Work out the finished part from the listing and answer in its coordinate system (mm). A direction names the side the tool comes from. Round coordinates to 2 decimals unless told otherwise and drop trailing zeros. Order: outer loops, then holes, each group sorted by start corner. A loop starts at its lowest first (then second) coordinate and runs counter-clockwise, first axis right, second up. Notation, with made-up numbers: (71, -30.75) - (124, -30.75) arc R24 ccw to (124, 0.25) - close; hole circle Ø10 at (10.5, -14). An arc over 180 degrees is marked (long way). Put each result on its own line as item: value.
Autodesk Inventor part; units mm, degrees
ref_plane "YZ Plane" through (0, 0, 0) normal (1, 0, 0) x (0, 1, 0)
ref_plane "XZ Plane" through (0, 0, 0) normal (0, 1, 0) x (-1, 0, 0)
ref_plane "XY Plane" through (0, 0, 0) normal (0, 0, 1) x (1, 0, 0)
sketch "Sketch1" plane through (0, 0, 0) normal (0, 1, 0) x (-1, 0, 0)
  line L0 (0, 0) -> (-127, 0)
  line L1 (-127, 0) -> (-127, -6.35)
  line L2 (-127, -6.35) -> (0, -6.35)
  line L3 (0, -6.35) -> (0, 0)
  line L4 (0, -6.35) -> (-6.35, -6.35)
  line L5 (-6.35, -6.35) -> (-6.35, -127)
  line L6 (-6.35, -127) -> (0, -127)
  line L7 (0, -127) -> (0, -6.35)
  line L8 (-127, -6.35) -> (-120.65, -6.35)
  line L9 (-120.65, -6.35) -> (-120.65, -127)
  line L10 (-120.65, -127) -> (-127, -127)
  line L11 (-127, -127) -> (-127, -6.35)
  dimension "d0" = 127
  dimension "d1" = 6.35
  dimension "d2" = 6.35
  dimension "d3" = 120.65
  dimension "d4" = 120.65
  dimension "d5" = 6.35
extrude "Extrusion1" add sketch "Sketch1" along normal blind 6.35
sketch "Sketch2" plane through (127, 0, 0) normal (1, 0, 0) x (0, 0, -1)
  line L0 (127, 6.35) -> (120.65, 0)
  line L1 (6.35, 0) -> (127, 0)
  line L2 (127, 0) -> (127, 6.35)
  line L3 (120.65, 0) -> (127, 0)
  line L4 (127, 0) -> (127, 6.35)
  line L5 (127, 6.35) -> (127, 0)
  point P0 (0, 0)
  dimension "d8" = 135
extrude "Extrusion2" cut sketch "Sketch2" against normal blind 152.4
sketch "Sketch4" plane through (0, 6.35, 0) normal (0, 1, 0) x (1, 0, 0)
  line L0 (127, 120.65) -> (127, 127)
  line L1 (127, 120.65) -> (127, 127)
  line L2 (127, 127) -> (120.65, 127)
  line L3 (120.65, 127) -> (120.65, 120.65)
  line L4 (120.65, 120.65) -> (127, 120.65)
  point P0 (0, 0)
extrude "Extrusion3" cut sketch "Sketch4" against normal blind 152.4
sketch "Sketch5" plane through (0, 6.35, 0) normal (0, 1, 0) x (1, 0, 0)
  line L0 (120.65, 120.65) -> (120.65, 127.0036)
  line L1 (120.65, 127.0036) -> (127.0123, 127.0036)
  line L2 (127.0123, 127.0036) -> (127.0123, 120.65)
  line L3 (127.0123, 120.65) -> (120.65, 120.65)
  point P0 (0, 0)
extrude "Extrusion4" add sketch "Sketch5" against normal blind 152.4
sketch "Sketch6" plane through (0, 6.35, 0) normal (0, 1, 0) x (1, 0, 0)
  line L0 (0, 127) -> (0, 120.65)
  line L1 (0, 127) -> (0, 120.65)
  line L2 (0, 120.65) -> (6.35, 120.65)
  line L3 (0, 120.65) -> (6.35, 120.65)
  line L4 (6.35, 120.65) -> (6.35, 127)
  line L5 (6.35, 127) -> (0, 127)
  point P0 (0, 0)
extrude "Extrusion5" cut sketch "Sketch6" against normal blind 101.6
sketch "Sketch7" plane through (0, 6.35, 0) normal (0, 1, 0) x (1, 0, 0)
  line L0 (0, 120.65) -> (6.35, 120.65)
  line L1 (6.35, 120.65) -> (6.35, 126.9915)
  line L2 (6.35, 126.9915) -> (0, 126.9915)
  line L3 (0, 126.9915) -> (0, 120.65)
  point P0 (0, 0)
extrude "Extrusion6" add sketch "Sketch7" against normal blind 152.4
sketch "Sketch8" plane through (6.35, 0, -6.35) normal (1, 0, 0) x (0, 0, -1)
  line L0 (120.6415, 6.35) -> (120.6415, -146.05)
  line L1 (114.3, -146.05) -> (120.6415, -146.05)
  line L2 (120.6415, -146.05) -> (120.6415, -139.7)
  line L3 (120.6415, -139.7) -> (114.3, -139.7)
  line L4 (114.3, -139.7) -> (114.3, -146.05)
  point P0 (-6.35, 0)
  dimension "d19" = 6.35
extrude "Extrusion7" add sketch "Sketch8" along normal blind 120.65
sketch "Sketch9" plane through (0, 6.35, 0) normal (0, 1, 0) x (1, 0, 0)
  line L0 (0, 126.9915) -> (127, 126.9915)
  line L1 (127, 126.9915) -> (127, 0)
  line L2 (127, 0) -> (0, 0)
  line L3 (0, 0) -> (0, 126.9915)
extrude "Extrusion8" add sketch "Sketch9" along normal blind 3.175
sketch "Sketch10" plane through (0, 9.525, 0) normal (0, 1, 0) x (1, 0, 0)
  circle A0 centre (31.75, 95.2415) radius 14.351
  circle A1 centre (95.25, 95.2415) radius 14.351
  circle A2 centre (31.75, 31.75) radius 14.351
  circle A3 centre (95.25, 31.75) radius 14.351
  line L0 (0, 126.9915) -> (0, 0)
  line L1 (127, 0) -> (127, 126.9915)
  line L2 (127, 126.9915) -> (0, 126.9915)
  line L3 (0, 0) -> (127, 0)
  dimension "d24" = 28.702
  dimension "d25" = 28.702
  dimension "d26" = 28.702
  dimension "d27" = 28.702
  dimension "d28" = 31.75
  dimension "d29" = 31.75
  dimension "d30" = 31.75
  dimension "d31" = 31.75
  dimension "d32" = 31.75
  dimension "d33" = 31.75
  dimension "d34" = 31.75
  dimension "d35" = 31.75
extrude "Extrusion9" cut sketch "Sketch10" against normal blind 25.4 contours A0 | A1 | A2 | A3
ref_plane "Work Plane1" through (0, 0, 0) normal (0, -0.6368859, 0.7709581) x (1, 0, 0)
sketch "Sketch12" plane through (127, 0, -120.65) normal (1, 0, 0) x (0, 0, -1)
  line L0 (6.3415, 9.525) -> (6.3536, -146.05)
  line L1 (6.3536, -146.05) -> (0, -146.05)
  line L2 (6.3536, -146.05) -> (0, -146.05)
  line L3 (0, -146.05) -> (-120.65, 0)
  line L4 (-120.65, 0) -> (-120.65, 9.525)
  line L5 (-120.65, 0) -> (-120.65, 9.525)
  line L6 (-120.65, 9.525) -> (6.3415, 9.525)
  line L7 (-120.65, 9.525) -> (6.3415, 9.525)
extrude "Extrusion11" add sketch "Sketch12" against normal blind 3.175
sketch "Sketch13" plane through (0, -146.05, -126.9915) normal (-1, 0, 0) x (0, 0, 1)
  line L0 (-0.0121, 0) -> (0, 155.575)
  line L1 (0, 155.575) -> (126.9915, 155.575)
  line L2 (126.9915, 155.575) -> (0, 155.575)
  line L3 (126.9915, 155.575) -> (126.9915, 146.05)
  line L4 (126.9915, 146.05) -> (6.3415, 0)
  line L5 (6.3415, 0) -> (126.9915, 146.05)
  line L6 (6.3415, 0) -> (-0.0121, 0)
extrude "Extrusion12" add sketch "Sketch13" against normal blind 3.175
sketch "Sketch15" plane through (0, 0, 0) normal (0, -0.6368859, 0.7709581) x (1, 0, 0)
  line L0 (127.0123, -189.4387) -> (0, -189.4387)
  line L1 (0, -189.4387) -> (0, 0)
  line L2 (0, 0) -> (127.0123, 0)
  line L3 (127.0123, 0) -> (127.0123, -189.4387)
extrude "Extrusion14" add sketch "Sketch15" along normal blind 25.4
sketch "Sketch16" plane through (0, 0, 0) normal (0, 0.6368859, -0.7709581) x (-1, 0, 0)
  line L0 (-6.35, 0.8514) -> (-120.65, 0.8514)
  line L1 (-120.65, 0.8514) -> (-120.65, -186.5598)
  line L2 (-120.65, -186.5598) -> (-6.35, -186.5598)
  line L3 (-6.35, -186.5598) -> (-6.35, 0.8514)
  point P0 (0, 0)
extrude "Extrusion15" cut sketch "Sketch16" against normal blind 22.225
sketch "Sketch17" plane through (0, -16.1769, 19.5823) normal (0, 0.7709581, 0.6368859) x (1, 0, 0)
  line L0 (127, 122.4603) -> (127, 25.4)
  line L1 (0, 0) -> (127, 0)
  line L2 (127, 0) -> (127, 31.3747)
  line L3 (127, 31.3747) -> (0, 31.3747)
  line L4 (0, 31.3747) -> (0, 0)
  point P0 (0, 25.4)
extrude "Extrusion16" add sketch "Sketch17" along normal blind 7.9375
fillet "Fillet1" radius 3.175 2 edges at (63.5, 9.525, 0) (63.5, 9.9247, 0.4491)
sketch "Sketch19" plane through (0, -146.05, -120.65) normal (0, -0.7709581, -0.6368859) x (1, 0, 0)
  line L0 (127, 25.3989) -> (0, 25.3989)
  line L1 (0, 25.3989) -> (0, -5.2114)
  line L2 (0, -5.2114) -> (127, -5.2114)
  line L3 (127, -5.2114) -> (127, 25.3989)
  point P0 (0, -0.0011)
extrude "Extrusion17" add sketch "Sketch19" along normal blind 3.9688
sketch "Sketch23" plane through (0, 9.525, 0) normal (0, 1, 0) x (1, 0, 0)
  line L0 (6.35, 118.8173) -> (120.65, 118.8173)
  line L1 (123.825, 126.9915) -> (3.175, 126.9915)
  circle A0 centre (63.5, 120.6415) radius 2.54
  line L2 (0, 126.9915) -> (0, 0.9451)
  line L3 (127, 0.9451) -> (127, 126.9915)
  point P0 (0, 0)
  dimension "d78" = 6.35
  dimension "d80" = 63.5
  dimension "d82" = 5.08
extrude "Extrusion21" cut sketch "Sketch23" against normal blind 7.62
properties part number "button_angle"
1) A cutting plane is placed at A-A on x = 35. Give the number of separate pieces and of enclosed holes in the cut face, then the cut area to 3 significant figures.
Findings below:
separate pieces: 3
enclosed holes: 0
area: 1,310 mm2
2) For a pull along X with two mould halves and no side action, classify faces 1 (the flat face through (64, 0, -2)), 2 (the flat face through (127, -154, -114)), 3 (the flat face through (0, -57, -69)) as pulls with the +X half, pulls with the -X half, needs draft (parallel to the pull), parting line crosses it, or undercut.
Findings below:
face 1: undercut
face 2: pulls with the +X half
face 3: pulls with the -X half
3) Straight lines are drawn through the part: L1, parallel to X at y = 7.8, z = -31.75; L2, parallel to X at y = -55, z = -107 (3 decimals); L3, parallel to Z at x = 95, y = 7. For each, find the intervals that lie inside material, in ascending order. Write a range as from..to.
Findings below:
L1: x = 0..17.4, 46.1..80.9, 109.6..127
L2: x = 0..3.175, 123.825..127
L3: z = -126.99..-109.59, -80.89..-46.1, -17.4..3.99
4) Given pin 1 Ø2 at (x, y) = (65.5, -60) entering from +Z; pin 2 Ø6 at (x, z) = (95, -14.5) entering from -Y; pin 3 Ø5 at (x, z) = (65, -124.5) entering from -Y, each flat-ended and moving along its own axis, determine where each tip first touches the part or whether it passes through.
Findings below:
pin 1: stops at z = -15.79
pin 2: stops at y = -61.07
pin 3: stops at y = -150.08
5) A cutting plane is placed at B-B on z = -31.75. Write down the section's boundary in (x, y) (3 decimals), then the cut area to 3 significant figures.
Findings below:
outline: (0, -78.315) - (127.012, -78.315) - (127.012, -38.434) - (127, -38.434) - (127, 9.525) - (109.601, 9.525) - (109.601, 6.35) - (120.65, 6.35) - (120.65, 0) - (123.825, 0) - (123.825, -38.434) - (120.65, -38.434) - (120.65, -73.333) - (6.35, -73.333) - (6.35, -38.434) - (3.175, -38.434) - (3.175, 0) - (6.35, 0) - (6.35, 6.35) - (17.399, 6.35) - (17.399, 9.525) - (0, 9.525) - close; (46.101, 6.35) - (80.899, 6.35) - (80.899, 9.525) - (46.101, 9.525) - close
area: 1,620 mm2
6) For faces 4 (the flat face through (63, -143, -120.65)), 5 (the flat face through (62.61, -0.57, 13.15)), 6 (the flat face through (120.65, -30, -124)), 7 (the cylindrical face through (45.44, 7.96, -36.06)), determine the directions among +Z, -Z, +X, -X, +Y, -Y from which every point of the face is accessible in a straight line to the end or side of a thin tool.
Findings below:
face 4: none
face 5: +Z, +X, -X, +Y
face 6: -Z
face 7: +Y
